```python
from build123d import *

# Parameters (mm, degrees)
SKETCH1_R           = 5.588
BOSS_EXTRUDE1_DEPTH = 2.286
BOSS_EXTRUDE2_DEPTH = 2.286
FILLET1_R           = 2.286
FILLET2_R           = 4.572


with BuildPart() as part:
    # Sketch1 → Boss-Extrude1 (new body)
    with BuildSketch(Plane.XY):
        with BuildLine():
            Line((-17.526, 0), (17.526, 0))
            Line((17.526, 0), (17.526, 3.048))
            Line((17.526, 3.048), (7.94015483, 16.917717675))
            ThreePointArc((7.94015483, 16.917717675), (0, 21.082), (-7.94015483, 16.917717675))
            Line((-7.94015483, 16.917717675), (-17.526, 3.048))
            Line((-17.526, 3.048), (-17.526, 0))
        make_face()
        with Locations((0, 14.224)):
            Circle(SKETCH1_R, mode=Mode.SUBTRACT)
    extrude(amount=BOSS_EXTRUDE1_DEPTH)

    # Sketch2 → Boss-Extrude2 (add)
    with BuildSketch(Plane(origin=(0, 0, 2.286), x_dir=(1, 0, 0), z_dir=(0, 1, 0))):
        with BuildLine():
            Line((-12.7, -4.953), (-17.526, -4.953))
            Line((-17.526, -4.953), (-17.526, 2.286))
            Line((-17.526, 2.286), (17.526, 2.286))
            Line((17.526, 2.286), (17.526, -4.953))
            Line((17.526, -4.953), (12.7, -4.953))
            ThreePointArc((12.7, -4.953), (10.287, -7.366), (12.7, -9.779))
            Line((12.7, -9.779), (17.526, -9.779))
            Line((17.526, -9.779), (17.526, -11.938))
            ThreePointArc((17.526, -11.938), (16.558866591, -14.272866591), (14.224, -15.24))
            Line((14.224, -15.24), (-14.224, -15.24))
            ThreePointArc((-14.224, -15.24), (-16.558866591, -14.272866591), (-17.526, -11.938))
            Line((-17.526, -11.938), (-17.526, -9.779))
            Line((-17.526, -9.779), (-12.7, -9.779))
            ThreePointArc((-12.7, -9.779), (-10.287, -7.366), (-12.7, -4.953))
        make_face()
    extrude(amount=BOSS_EXTRUDE2_DEPTH)

    # Fillet1
    fillet1_edges = [part.edges().sort_by_distance(p)[0] for p in [
        (0, 2.286, 2.286),
    ]]
    fillet(fillet1_edges, radius=FILLET1_R)

    # Fillet2
    fillet2_edges = [part.edges().sort_by_distance(p)[0] for p in [
        (0, 0, 0),
    ]]
    fillet(fillet2_edges, radius=FILLET2_R)


solid = part.part
```
Input: part model. Units: mm. Frame: model coordinates. A direction names the side the tool comes from. Round coordinates to 2 decimals unless told otherwise and drop trailing zeros. Loops run counter-clockwise (first coordinate to the right, second up) from the corner with the lowest first, then second, coordinate; pieces in that order, holes last. Notation, with made-up numbers: (34, 13) - (81, 13) arc R11 cw to (81, 30) - close; hole circle Ø10 at (66, 22). An arc over 180 degrees is marked (long way). One line per item, written item: value. Start each with the question number.
(1) Ray query, line 1 (Y direction, x = 1, z = 9.5); line 2 (Y direction, x = 0, z = 0.95). Return the intervals inside material, ascending. Write a range as [from, to].
(2) Section A-A, the plane x = 0. Return loops of the section in (y, z), plus the area to 3 significant figures.
(3) Section B-B, the plane y = 12.5. Return loops of the section in (x, z).
(4) Section C-C, the plane z = 6. Return loops of the section in (x, y), plus the area to 3 significant figures.
(5) Draft query along X for faces 5 (the cylindrical face through (-10.288, 1.127, 9.705)), 6 (the cylindrical face through (-0.727, 19.764, 1.127)), 7 (the cylindrical face through (0.25, 2.94, 2.97)). Return one class per face: +X half, -X half, draft (parallel to the pull), parting line (faces both ways), or undercut.
(6) Access query for faces 1 (the flat face through (15, 1, 7.239)), 2 (the flat face through (-15, 1, 12.065)), 3 (the flat face through (0, 7, 2.286)), 4 (the flat face through (-17.526, 2, 4)). Directions: +Z, -Z, +X, -X, +Y, -Y. A direction counts if a zero-diameter tool reaches every point of the face in a straight line with its end or side. Return the directions, or none.
(7) Section D-D, the plane y = 18.5. Return loops of the section in (x, z).
(8) Contact query for flat-ended pins moving along their axis: P1, Ø0.7, axis at x = -14.5, y = 1.5, coming from the -Z side; P2, Ø1.1, axis at x = 16, y = 1, coming from the -Z side; P3, Ø1.1, axis at x = -15.5, y = 0.5, coming from the +Z side. Output: stop coordinate, or through.
Results below:
1. line 1: [0, 2.29]
1. line 2: [1.78, 8.64], [19.81, 21.08]
2. outline: (0, 4.57) arc R4.57 ccw to (4.57, 0) - (8.64, 0) - (8.64, 2.29) - (4.57, 2.29) arc R2.29 cw to (2.29, 4.57) - (2.29, 17.53) - (0, 17.53) - close; (19.81, 0) - (21.08, 0) - (21.08, 2.29) - (19.81, 2.29) - close
2. area: 54.1 mm^2
3. outline: (-10.99, 0) - (-5.32, 0) - (-5.32, 2.29) - (-10.99, 2.29) - close; (5.32, 0) - (10.99, 0) - (10.99, 2.29) - (5.32, 2.29) - close
4. outline: (-17.53, 0) - (17.53, 0) - (17.53, 2.29) - (-17.53, 2.29) - close
4. area: 80.1 mm^2
5. face 5: -X half
5. face 6: undercut
5. face 7: draft
6. face 1: +X, +Y, -Y
6. face 2: -X, +Y, -Y
6. face 3: +Z, +X, -X, +Y
6. face 4: +Z, -Z, -X, +Y, -Y
7. outline: (-6.57, 0) - (-3.6, 0) - (-3.6, 2.29) - (-6.57, 2.29) - close; (3.6, 0) - (6.57, 0) - (6.57, 2.29) - (3.6, 2.29) - close
8. P1: z = 0.9
8. P2: z = 1.14
8. P3: z = 17.45
